Geometry check sheet. Reference: the model listing, model coordinates, mm. A direction names the side the tool comes from. Give positions to 0.01 mm unless a question says otherwise; leave off trailing zeros. Order: outer loops, then holes, each group sorted by start corner. A loop starts at its lowest first (then second) coordinate and runs counter-clockwise, first axis right, second up.
from build123d import *

# Parameters (mm, degrees)
SKETCH1_R           = 2.5
SKETCH1_R_2         = 1.25
BOSS_EXTRUDE1_DEPTH = 1
SKETCH2_W           = 15
SKETCH2_H           = 10
SKETCH2_R           = 2
BOSS_EXTRUDE2_DEPTH = 1
FILLET1_R           = 2


with BuildPart() as part:
    # Sketch1 → Boss-Extrude1 (new, symmetric)
    with BuildSketch(Plane.XY):
        with BuildLine():
            Line((0, 5), (20, 5))
            ThreePointArc((20, 5), (25, 0), (20, -5))
            Line((20, -5), (0, -5))
            ThreePointArc((0, -5), (-5, 0), (0, 5))
        make_face()
        Circle(SKETCH1_R, mode=Mode.SUBTRACT)
        with Locations((20, 0)):
            Circle(SKETCH1_R, mode=Mode.SUBTRACT)
        with Locations((10, -3)):
            Circle(SKETCH1_R_2, mode=Mode.SUBTRACT)
    extrude(amount=BOSS_EXTRUDE1_DEPTH, both=True)

    # Sketch2 → Boss-Extrude2 (add, symmetric)
    with BuildSketch(Plane.XY):
        with Locations((10, 10)):
            Rectangle(SKETCH2_W, SKETCH2_H)
        with Locations((10, 9.5)):
            Circle(SKETCH2_R, mode=Mode.SUBTRACT)
    extrude(amount=BOSS_EXTRUDE2_DEPTH, both=True)

    # Fillet1
    fillet1_edges = [part.edges().sort_by_distance(p)[0] for p in [
        (2.5, 15, 0),
        (17.5, 15, 0),
    ]]
    fillet(fillet1_edges, radius=FILLET1_R)


solid = part.part
Item 1: Scan lines: L1, parallel to Y at x = 10, z = 0.05; L2, parallel to X at y = -3.5, z = 0.75; L3, parallel to Y at x = 20, z = 0.3. Record each from-to range of solid material in increasing order.
Reported:
L1: y = -5 to -4.25, -1.75 to 7.5, 11.5 to 15
L2: x = -3.57 to 8.85, 11.15 to 23.57
L3: y = -5 to -2.5, 2.5 to 5
Item 2: Draft check along X on faces 1 (the cylindrical face through (-5, 0, 0)), 2 (the cylindrical face through (17.5, 0.1, 0)), 3 (the flat face through (19, 5, 0)), 4 (the cylindrical face through (16.9, 14.43, -0.01)). Enter one of: released by +X, released by -X, zero draft, split by the parting line, or undercut.
Reported:
face 1: released by -X
face 2: undercut
face 3: zero draft
face 4: released by +X
Item 3: Sectioned sample at A-A (y = 0). Enter the section's corners in (x, z), and give its area (3 significant figures).
Reported:
outline: (-5, -1) - (-2.5, -1) - (-2.5, 1) - (-5, 1) - close; (2.5, -1) - (17.5, -1) - (17.5, 1) - (2.5, 1) - close; (22.5, -1) - (25, -1) - (25, 1) - (22.5, 1) - close
area: 40.0 mm2
Item 4: Sectioned sample at C-C (z = -0.35). Enter the section's corners in (x, y), and give its area (3 significant figures).
Reported:
outline: (0, -5) - (20, -5) arc R5 ccw to (20, 5) - (17.5, 5) - (17.5, 13) arc R2 ccw to (15.5, 15) - (4.5, 15) arc R2 ccw to (2.5, 13) - (2.5, 5) - (0, 5) arc R5 ccw to start; hole circle Ø5 at (0, 0); hole circle Ø4 at (10, 9.5); hole circle Ø2.5 at (10, -3); hole circle Ø5 at (20, 0)
area: 370 mm2
Item 5: Sectioned sample at D-D (y = -3). Enter the section's corners in (x, z), and give its area (3 significant figures).
Reported:
outline: (-4, -1) - (8.75, -1) - (8.75, 1) - (-4, 1) - close; (11.25, -1) - (24, -1) - (24, 1) - (11.25, 1) - close
area: 51.0 mm2
Item 6: Set-up check for faces 5 (the flat face through (17.5, 9, 0)), 6 (the flat face through (10, 5, -1)), 7 (the flat face through (1, 5, 0)): record each of +Z, -Z, +X, -X, +Y, -Y from which the full face is reachable in a straight line by a thin tool's end or side.
Reported:
face 5: +Z, -Z, +X, +Y
face 6: -Z, +X, -X, +Y, -Y
face 7: +Z, -Z, -X, +Y
Item 7: Gauge pin test, flat ends, axial feed: pin 1 (6 mm diameter, centred on x = 20, y = 0, fed in from +Z); pin 2 (3.5 mm diameter, centred on x = 10, y = 9.5, fed in from -Z); pin 3 (0.6 mm diameter, centred on y = 7.5, z = 0, fed in from -X); pin 4 (1 mm diameter, centred on y = 11, z = 0.5, fed in from +X). Record the tip position at first contact, or that the pin passes through.
Reported:
pin 1: stops at z = 1
pin 2: passes through
pin 3: stops at x = 2.5
pin 4: stops at x = 17.5
Item 8: Sectioned sample at B-B (x = 10). Enter the section's corners in (y, z), and give its area (3 significant figures).
Reported:
outline: (-5, -1) - (-4.25, -1) - (-4.25, 1) - (-5, 1) - close; (-1.75, -1) - (7.5, -1) - (7.5, 1) - (-1.75, 1) - close; (11.5, -1) - (15, -1) - (15, 1) - (11.5, 1) - close
area: 27.0 mm2
